Input: dimensioned drawing with shaded views. Units: mm. Origin: part minimum x, y, z. A direction names the side the tool comes from. Give positions to 0.01 mm unless a question says otherwise; leave off trailing zeros. Loops run counter-clockwise (first coordinate to the right, second up) from the corner with the lowest first, then second, coordinate; pieces in that order, holes last. Notation, with made-up numbers: (-18.75, 40) -> (-0.75, 40) arc R19 cw to (-0.75, 45) -> close; hole circle Ø9 at (-1, -23.5). An arc over 180 degrees is marked (long way). Answer as a JSON object with one key per item and string values.
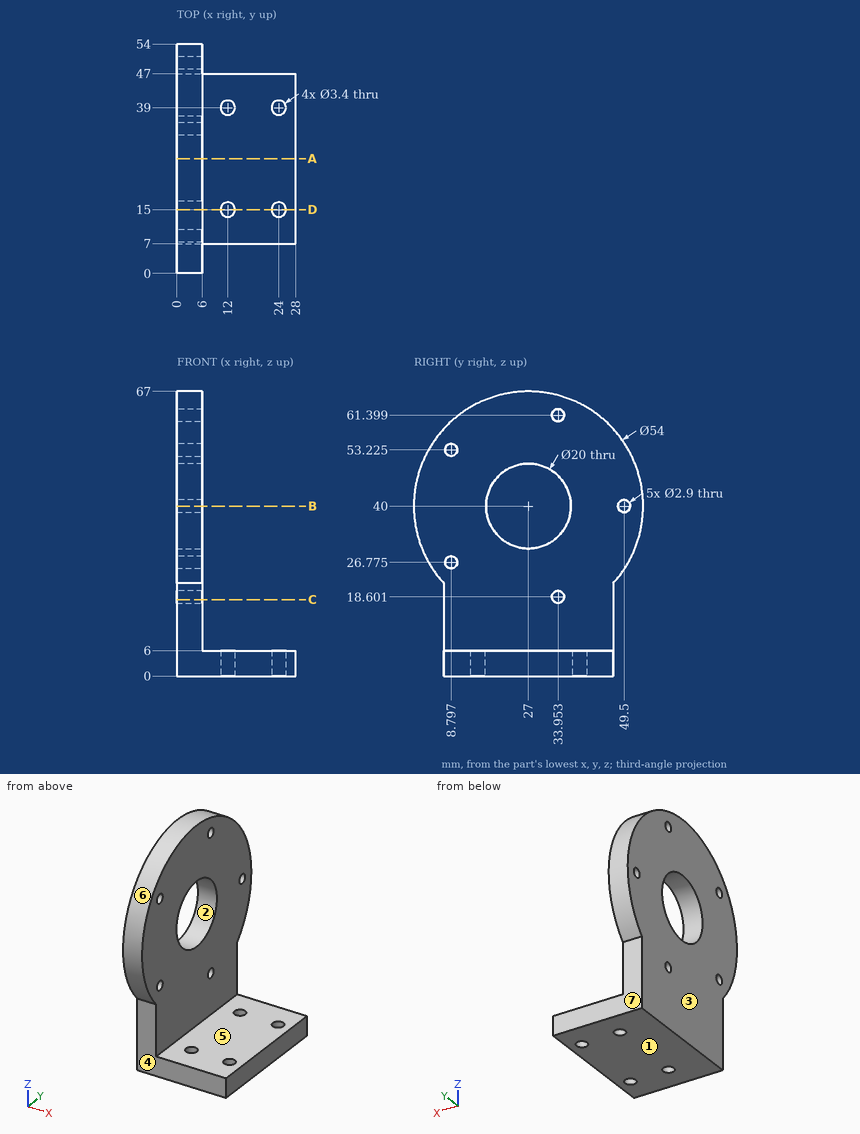
Q1. Pin query (flat end, axial travel): pin 1 (11 mm diameter, centred on x = 15.5, z = 11, fed in from -Y); pin 2 (8 mm diameter, centred on x = 18.5, y = 28.5, fed in from +Z); pin 3 (3.5 mm diameter, centred on y = 49.5, z = 40, fed in from +X). Return the tip coordinate at first contact, or that it passes through.
Evaluation:
{"pin 1": "stops at y = 7", "pin 2": "stops at z = 6", "pin 3": "stops at x = 6"}
Q2. Ray query, line 1 along X through (y, z) = (15, 2.7); line 2 along Z through (x, y) = (2.75, 33) (1 decimal); line 3 along Z through (x, y) = (19, 37). Return the intervals inside material, ascending.
Evaluation:
{"line 1": "x = 0 to 10.3, 13.7 to 22.3, 25.7 to 28", "line 2": "z = 0 to 17.5, 19.7 to 32, 48 to 60.3, 62.5 to 66.3", "line 3": "z = 0 to 6"}
Q3. Section B-B, the plane z = 40. Return the cut outline in (x, y), then the cut area to 3 significant figures.
Evaluation:
{"outline": "(0, 0) -> (6, 0) -> (6, 17) -> (0, 17) -> close; (0, 37) -> (6, 37) -> (6, 48.05) -> (0, 48.05) -> close; (0, 50.95) -> (6, 50.95) -> (6, 54) -> (0, 54) -> close", "area": "187 mm2"}
Q4. Draft query along Z for the marked faces 1, 2 and 3. Return one class per face: +Z half, -Z half, draft (parallel to the pull), parting line (faces both ways), or undercut.
Evaluation:
{"face 1": "-Z half", "face 2": "undercut", "face 3": "draft"}
Q5. Section D-D, the plane y = 15. Return the cut outline in (x, z), then the cut area to 3 significant figures.
Evaluation:
{"outline": "(0, 0) -> (10.3, 0) -> (10.3, 6) -> (6, 6) -> (6, 64.19) -> (0, 64.19) -> close; (13.7, 0) -> (22.3, 0) -> (22.3, 6) -> (13.7, 6) -> close; (25.7, 0) -> (28, 0) -> (28, 6) -> (25.7, 6) -> close", "area": "476 mm2"}
Q6. Access query for the marked faces 4, 5, 6 and 7. Directions: +Z, -Z, +X, -X, +Y, -Y. A direction counts if a zero-diameter tool reaches every point of the face in a straight line with its end or side. Return the directions, or none.
Evaluation:
{"face 4": "-Z, +X, -X, -Y", "face 5": "+Z, +X, +Y, -Y", "face 6": "+X, -X", "face 7": "-Z, +X, -X, +Y"}
Q7. Section C-C, the plane z = 18. Return the cut outline in (x, y), then the cut area to 3 significant figures.
Evaluation:
{"outline": "(0, 7) -> (6, 7) -> (6, 32.63) -> (0, 32.63) -> close; (0, 35.27) -> (6, 35.27) -> (6, 47) -> (0, 47) -> close", "area": "224 mm2"}
Q8. Section A-A, the plane y = 27. Return the cut outline in (x, z).
Evaluation:
{"outline": "(0, 0) -> (28, 0) -> (28, 6) -> (6, 6) -> (6, 30) -> (0, 30) -> close; (0, 50) -> (6, 50) -> (6, 67) -> (0, 67) -> close"}
